Check sheet for the modelled part. Datum: model origin and axes. Units: mm. Give positions to 0.01 mm unless a question says otherwise; leave off trailing zeros. Order: outer loops, then holes, each group sorted by start corner. A loop starts at its lowest first (then second) coordinate and runs counter-clockwise, first axis right, second up. Notation, with made-up numbers: M 49.5,46.5 L 97.5,46.5 A21 ccw 97.5,69.5 Z; hole C 61.5,9 d3. An arc over 180 degrees is marked long. Answer in a Markdown table with one row per item. Add a question column.
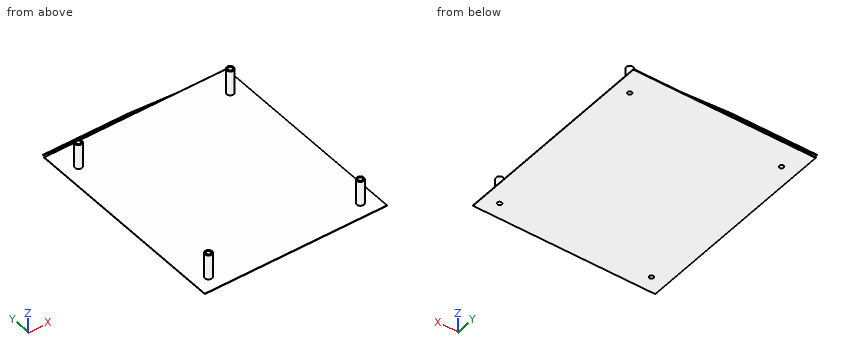
Autodesk Inventor part; units mm, degrees
ref_plane "YZ Plane" through (0, 0, 0) normal (1, 0, 0) x (0, 1, 0)
ref_plane "XZ Plane" through (0, 0, 0) normal (0, 1, 0) x (-1, 0, 0)
ref_plane "XY Plane" through (0, 0, 0) normal (0, 0, 1) x (1, 0, 0)
sketch "Sketch1" plane through (0, 0, 0) normal (0, 0, 1) x (1, 0, 0)
  line L0 (-90, -105) -> (90, -105)
  line L1 (90, -105) -> (90, 105)
  line L2 (-90, 105) -> (-90, -105)
  line L3 (42, 105) -> (42, 105)
  line L4 (42, 105) -> (-42, 105)
  line L5 (-42, 105) -> (-42, 105)
  line L6 (90, 105) -> (42, 105)
  line L7 (-42, 105) -> (-90, 105)
  point P0 (0, 0)
  dimension "d0" = 180
  dimension "d1" = 210
  dimension "d2" = 105
  dimension "d3" = 90
  dimension "d22" = 0
  dimension "d24" = 42
  dimension "d26" = 84
  dimension "d28" = 0
  dimension "d29" = 210
  dimension "d30" = 48
  dimension "d31" = 48
extrude "Plate1" add sketch "Sketch1" along normal blind 0.5
sketch "Sketch6" plane through (90, 104.6464, 0.1464) normal (0, 0.7071068, 0.7071068) x (-1, 0, 0)
  line L0 (180, 0) -> (0, 0)
  line L1 (0, 0) -> (0, -92)
  line L2 (0, -92) -> (180, -92)
  line L3 (180, -92) -> (180, 0)
edge flange "Flange1" height 92 angle 45 thickness 0.5 bend radius 0.5 thickness toward (0, 0.7071068, 0.7071068) relief tear relief width 0.5 relief depth 0.25 edges at (66, 105, 0) wall of the first edge with corners at (-90, 104.6464, 0.1464) (90, 104.6464, 0.1464) (90, 169.7003, -64.9074) (-90, 169.7003, -64.9074)
bend "Bend1"
corner "Corner1"
sketch "Sketch7" plane through (90, 169.7003, -64.9074) normal (0, -0.7071068, -0.7071068) x (-1, 0, 0)
  line L0 (180, 0) -> (0, 0)
  line L1 (180, -91.9393) -> (0, -91.9393)
  line L2 (180, -91.5858) -> (180, 0)
  line L3 (0, -91.5858) -> (0, 0)
  line L4 (0, -91.5858) -> (180, -91.5858)
  line L5 (0, -91.5858) -> (180, -91.5858)
  line L6 (180, -91.5858) -> (180, 0)
  line L7 (180, 0) -> (0, 0)
  line L8 (0, -91.5858) -> (0, 0)
  line L9 (0, -91.5858) -> (48, -91.5858)
  line L10 (48, -91.5858) -> (48, 0)
  line L11 (48, 0) -> (0, 0)
  line L12 (0, 0) -> (0, -91.5858)
  point P0 (90, -165.8927)
  dimension "d88" = 180
  dimension "d89" = 48
extrude "Extrusion4" cut sketch "Sketch7" against normal blind 10 contours L10 L4 L3 L0
mirror "Mirror1" about plane through (0, 0, 0) normal (1, 0, 0) of "Extrusion4"
sketch "Sketch8" plane through (42, 169.7003, -64.9074) normal (0, -0.7071068, -0.7071068) x (-1, 0, 0)
  line L0 (81, -3) -> (3, -3)
  line L1 (3, -3) -> (3, -81)
  line L2 (3, -81) -> (81, -81)
  line L3 (81, -81) -> (81, -3)
  line L4 (81, -3) -> (3, -81) construction
  line L5 (3, -3) -> (81, -81) construction
  line L6 (84, 0) -> (0, 0)
  point P0 (42, -165.8927)
  point P1 (42, -42)
  dimension "d92" = 78
  dimension "d93" = 0
  dimension "d94" = 3
  dimension "d111" = 78
extrude "Extrusion5" cut sketch "Sketch8" against normal blind 10
chamfer "Chamfer2" distance 16 angle 45 4 edges at (39, 112.6014, -7.455) (39, 167.7557, -62.6093) (-39, 167.7557, -62.6093) (-39, 112.6014, -7.455)
sketch "Sketch9" plane through (42, 169.7003, -64.9074) normal (0, -0.7071068, -0.7071068) x (-1, 0, 0)
  line L0 (77.75, -5) -> (6.25, -5) construction
  line L1 (6.25, -5) -> (6.25, -76.5) construction
  line L2 (6.25, -76.5) -> (77.75, -76.5) construction
  line L3 (77.75, -76.5) -> (77.75, -5) construction
  line L4 (77.75, -5) -> (6.25, -76.5) construction
  line L5 (6.25, -5) -> (77.75, -76.5) construction
  line L6 (84, 0) -> (0, 0) construction
  point P0 (42, -165.8927)
  point P1 (42, -40.75)
  dimension "d100" = 71.5
  dimension "d101" = 71.5
  dimension "d102" = 35.75
  dimension "d103" = 5
hole "Hole3" at (35.75, 166.1647, -61.3718) at (-35.75, 166.1647, -61.3718) at (-35.75, 115.6066, -10.8137) at (35.75, 115.6066, -10.8137) direction (0, 0.7071068, 0.7071068) diameter 4.2 end through all
sketch "Sketch10" plane through (0, 0, 0) normal (0, 0, -1) x (-1, 0, 0)
  line L0 (-75, -90) -> (75, -90) construction
  line L1 (75, -90) -> (75, 80) construction
  line L2 (75, 80) -> (-75, 80) construction
  line L3 (-75, 80) -> (-75, -90) construction
  line L4 (-75, -90) -> (75, 80) construction
  line L5 (75, -90) -> (-75, 80) construction
  line L6 (90, -105) -> (-90, -105)
  point P0 (0, -5)
  point P1 (0, 0)
  dimension "d112" = 170
  dimension "d113" = 150
  dimension "d114" = 75
  dimension "d115" = 15
hole "Hole4" at (75, 80, 0) at (75, -90, 0) at (-75, -90, 0) at (-75, 80, 0) direction (0, 0, 1) diameter 4.2 end through all
sketch "Sketch11" plane through (0, 0, 0) normal (0, 0, -1) x (-1, 0, 0)
  circle A0 centre (-75, 80) radius 2.1
  circle A1 centre (-75, 80) radius 3.5
  circle A2 centre (-75, -90) radius 2.1
  circle A3 centre (75, -90) radius 2.1
  circle A4 centre (75, 80) radius 2.1
  circle A5 centre (-75, -90) radius 3.5
  circle A6 centre (75, -90) radius 3.5
  circle A7 centre (75, 80) radius 3.5
  point P0 (0, 0)
  dimension "d123" = 7
  dimension "d124" = 7
  dimension "d125" = 7
  dimension "d126" = 7
extrude "Extrusion7" add sketch "Sketch11" against normal blind 25
equation "\"d111\" = d92"
equation "\"d101\" = d100"
equation "\"d109\" = Thickness"
equation "\"d121\" = Thickness"
equation "\"d74\" = Thickness"
equation "\"d75\" = BendReliefWidth"
equation "\"d76\" = BendReliefDepth"
equation "\"d77\" = MinimumRemnant"
equation "\"d78\" = TransitionRadius"
equation "\"d81\" = BendRadius"
equation "\"d82\" = CornerReliefSize"
equation "\"d83\" = GapSize"
equation "\"d84\" = JacobiRadiusSize"
equation "\"BendRadius\" = Thickness"
equation "\"BendReliefWidth\" = Thickness"
equation "\"BendReliefDepth\" = 0.5 * Thickness"
equation "\"CornerReliefSize\" = 4 * Thickness"
equation "\"MinimumRemnant\" = 2 * Thickness"
equation "\"TransitionRadius\" = BendRadius"
equation "\"JacobiRadiusSize\" = BendRadius"
equation "\"GapSize\" = Thickness"
properties part number "XGEN_hotbed-pcb"
Q1. Cross-section at C-C (x = 66.5). Record the boundary of the cut face in (y, z), and give its area (3 significant figures).
Q2. Cross-section at B-B (y = 145.5). Record the boundary of the cut face in (x, z), and give its area (3 significant figures).
Q3. Cross-section at A-A (z = -25). Record the boundary of the cut face in (x, y).
Q4. Go/stop test with flat-tipped pins: pin 1 (6 mm diameter, centred on x = -25.5, y = -47.5, fed in from +Z); pin 2 (6.5 mm diameter, centred on x = -75, y = 80, fed in from -Z); pin 3 (10 mm diameter, centred on y = 143.5, z = -42.5, fed in from -X). Record where each tip stops, or that it passes through.
Q5. Thickness scan on probe 1 along Y at (x, z) = (75, 14); probe 2 along Z at (x, y) = (14, -3.5); probe 3 along Y at (x, z) = (-41, -22.5). Record the ranges inside material, lowest first.
Q6. Cross-section at D-D (y = 28). Record the boundary of the cut face in (x, z), and give its area (3 significant figures).
Values follow:
| question | item | result |
|---|---|---|
| 1 | outline | M -105,0 L 104.59,0 A0.5 cw 104.94,-0.15 L 105.29,0.21 A1 ccw 104.59,0.5 L -105,0.5 Z |
| 1 | area | 105 mm² |
| 2 | outline | M -42,-40.71 L -39,-40.71 L -39,-40 L -42,-40 Z; M 39,-40.71 L 42,-40.71 L 42,-40 L 39,-40 Z |
| 2 | area | 4.24 mm² |
| 3 | outline | M -42,129.79 L -39,129.79 L -39,130.5 L -42,130.5 Z; M 39,129.79 L 42,129.79 L 42,130.5 L 39,130.5 Z |
| 4 | pin 1 | z = 0.5 |
| 4 | pin 2 | z = 0 |
| 4 | pin 3 | x = -42 |
| 5 | probe 1 | -93.5 to -92.1, -87.9 to -86.5, 76.5 to 77.9, 82.1 to 83.5 |
| 5 | probe 2 | 0 to 0.5 |
| 5 | probe 3 | 127.29 to 128 |
| 6 | outline | M -90,0 L 90,0 L 90,0.5 L -90,0.5 Z |
| 6 | area | 90.0 mm² |
